The listing builds one solid part. Answer for the finished solid, in the listing's coordinates (mm). Face numbers are marked on the shaded views. A direction names the side the tool comes from. Round coordinates to 2 decimals unless told otherwise and drop trailing zeros. Write each loop counter-clockwise with the first axis right and the second up, starting at its lowest first coordinate (ties: lowest second). Pieces come first, ordered by that corner, then holes. Notation, with made-up numbers: (-6.75, -11.5) - (7.25, -11.5) arc R30 ccw to (7.25, 11.5) - close; hole circle Ø7 at (84.5, -20). An arc over 180 degrees is marked (long way). Answer as CSV lines item,"result". Start each with the question number.
Item 1: A cutting plane is placed at B-B on z = -5. Determine the outline of the cut face in (x, y).
Item 2: For a pull along Z with two mould halves and no side action, classify the marked faces 3, 4 and 5 as pulls with the +Z half, pulls with the -Z half, needs draft (parallel to the pull), parting line crosses it, or undercut.
Item 3: Which of the six approach directions +Z, -Z, +X, -X, +Y, -Y give full straight-line access (tool end or side, diameter ignored) to the marked faces 1 and 2?
Item 4: Straight lines are drawn through the part: line 1 along Z through (x, y) = (3.75, 1.85); line 2 along X through (y, z) = (0.2, -1.75); line 3 along Z through (x, y) = (2.25, 0.85). For each, find the intervals that lie inside material, in ascending order. Write a range as [from, to].
Item 5: A cutting plane is placed at A-A on y = 0.2. Determine the outline of the cut face in (x, z), and give its area (3 significant figures).
Item 6: A cutting plane is placed at C-C on x = 3.75. Determine the outline of the cut face in (y, z), and give its area (3 significant figures).
```python
from build123d import *

# Parameters (mm, degrees)
SKETCH1_W           = 8
SKETCH1_H           = 7
BOSS_EXTRUDE1_DEPTH = 2


with BuildPart() as part:
    # Sketch1 → Boss-Extrude1 (new body)
    with BuildSketch(Plane(origin=(0, 0, 0), x_dir=(1, 0, 0), z_dir=(0, 1, 0))):
        with Locations((4, 3.5)):
            Rectangle(SKETCH1_W, SKETCH1_H)
        Polygon((7.117691454, 3.5), (5.558845727, 6.2), (2.441154273, 6.2), (0.882308546, 3.5), (2.441154273, 0.8), (5.558845727, 0.8), align=None, mode=Mode.SUBTRACT)
    extrude(amount=BOSS_EXTRUDE1_DEPTH)


solid = part.part
```
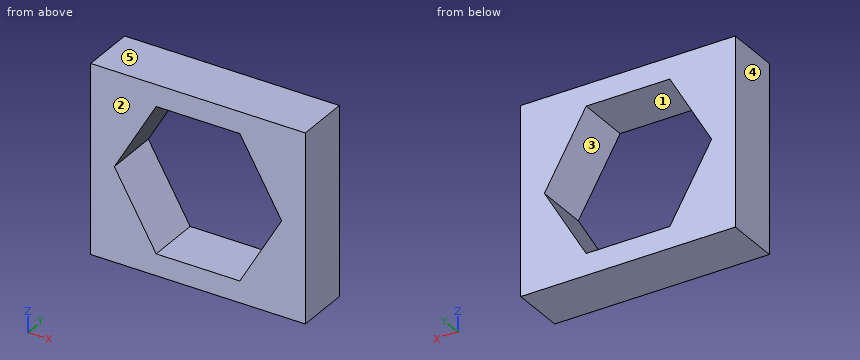
Geometry says:
1,outline,"(0, 0) - (1.75, 0) - (1.75, 2) - (0, 2) - close; (6.25, 0) - (8, 0) - (8, 2) - (6.25, 2) - close"
2,face 3,"undercut"
2,face 4,"needs draft"
2,face 5,"pulls with the +Z half"
3,face 1,"+Y, -Y"
3,face 2,"+Z, -Z, +X, -X, -Y"
4,line 1,"z = [-7, -6.2], [-0.8, 0]"
4,line 2,"x = [0, 1.89], [6.11, 8]"
4,line 3,"z = [-7, -5.87], [-1.13, 0]"
5,outline,"(0, -7) - (8, -7) - (8, 0) - (0, 0) - close; hole (0.88, -3.5) - (2.44, -6.2) - (5.56, -6.2) - (7.12, -3.5) - (5.56, -0.8) - (2.44, -0.8) - close"
5,area,"30.7 mm^2"
6,outline,"(0, -7) - (2, -7) - (2, -6.2) - (0, -6.2) - close; (0, -0.8) - (2, -0.8) - (2, 0) - (0, 0) - close"
6,area,"3.20 mm^2"
